```python
from build123d import *

# Parameters (mm, degrees)
SKETCH_R     = 7.85
PAD_DEPTH    = 4
FILLET_R     = 1.85
CHAMFER_SIZE = 1


with BuildPart() as part:
    # Sketch → Pad (new body)
    with BuildSketch(Plane.XY):
        with BuildLine():
            ThreePointArc((-11.001607, 0), (-0.009069, -10.999997), (10.998383, -0.014925))
            Line((15.968624, 10.800985), (10.998383, -0.014925))
            ThreePointArc((15.968624, 10.800985), (15.865486, 12.279709), (14.564905, 12.990872))
            Line((-14.567237, 12.990872), (14.564905, 12.990872))
            ThreePointArc((-14.567237, 12.990872), (-15.866325, 12.280427), (-15.969093, 10.803336))
            Line((-11.001607, 0), (-15.969093, 10.803336))
        make_face()
        Circle(SKETCH_R, mode=Mode.SUBTRACT)
    extrude(amount=PAD_DEPTH)

    # Fillet
    fillet_edges = [part.edges().sort_by_distance(p)[0] for p in [
        (-7.85, 0, 4),
        (-7.85, 0, 0),
    ]]
    fillet(fillet_edges, radius=FILLET_R)

    # Chamfer
    chamfer_edges = [part.edges().sort_by_distance(p)[0] for p in [
        (15.968624, 10.800985, 2),
        (13.483504, 5.39303, 4),
        (15.865486, 12.279709, 4),
        (-0.001166, 12.990872, 4),
        (-15.866325, 12.280427, 4),
        (-13.48535, 5.401668, 4),
        (-0.009069, -10.999997, 4),
        (-9.7, 0, 4),
        (-0.009069, -10.999997, 0),
        (13.483504, 5.39303, 0),
        (15.865486, 12.279709, 0),
        (-0.001166, 12.990872, 0),
        (-13.48535, 5.401668, 0),
    ]]
    chamfer(chamfer_edges, length=CHAMFER_SIZE)


solid = part.part
```
Work out the finished part from the listing and answer in its coordinate system (mm). Round coordinates to 2 decimals unless told otherwise and drop trailing zeros. Loops run counter-clockwise (first coordinate to the right, second up) from the corner with the lowest first, then second, coordinate; pieces in that order, holes last. Notation, with made-up numbers: (-28.5, -31.75) -> (-3.5, -31.75) arc R26 cw to (-3.5, -11.75) -> close; hole circle Ø2 at (-19, 78.5). An arc over 180 degrees is marked (long way). Write each question's results on one line, items separated by ' | '. Start each with the question number.
1. Section A-A (z = 0.6) is taken. Determine the outline of the cut face in (x, y).
2. Given pin 1 Ø2 at (x, y) = (2.5, 8) entering from -Z; pin 2 Ø2 at (y, z) = (-2.5, 2.5) entering from +X; pin 3 Ø3 at (x, y) = (7, 5) entering from +Z; pin 4 Ø2 at (y, z) = (4.5, 2.5) entering from +X, each flat-ended and moving along its own axis, determine where each tip first touches the part or whether it passes through.
3. Find the intervals of material crossed by probe 1 along Y at (x, z) = (0, 2); probe 2 along X at (y, z) = (2.75, 1.4); probe 3 along Y at (x, z) = (7, 1.7), in increasing order. Write a range as from..to.
4. Section B-B (x = 13.5) is taken. Determine the outline of the cut face in (y, z), plus the area to 3 significant figures.
Evaluation:
1) outline: (-15.61, 10.97) -> (-10.6, 0.09) arc R10.6 ccw (long way) to (10.6, 0.07) -> (15.61, 10.97) arc R1.14 ccw to (14.56, 12.59) -> (-14.57, 12.59) arc R1.14 ccw to start; hole circle Ø16.67 at (0, 0)
2) pin 1: stops at z = 0.03 | pin 2: stops at x = 10.9 | pin 3: stops at z = 4 | pin 4: stops at x = 13.53
3) probe 1: y = -11..-7.85, 7.85..12.99 | probe 2: x = -12.27..-7.41, 7.41..12.27 | probe 3: y = -8.48..-3.57, 3.57..12.99
4) outline: (5.43, 1) -> (7.82, 0) -> (11.99, 0) -> (12.99, 1) -> (12.99, 3) -> (11.99, 4) -> (7.82, 4) -> (5.43, 3) -> close | area: 26.9 mm2
